The model under review builds one solid part; all positions refer to its coordinate system, in mm. Face numbers are marked on the shaded views. A direction names the side the tool comes from. Coordinates: 2 decimals unless noted, no trailing zeros. Write each loop counter-clockwise with the first axis right and the second up, starting at its lowest first coordinate (ties: lowest second). Pieces come first, ordered by that corner, then holes. Notation, with made-up numbers: (14, 60) - (54, 60) arc R18 ccw to (54, 71) - close; hole circle Ø1 at (72, -37.5). An arc over 180 degrees is marked (long way). Return JSON: item names as keys, results as strings. Group by question number.
(1) We need section D-D on z = 18. State the section outline as (x, y) points, then the cut area to 3 significant figures.
(2) We need section B-B on y = -6. State the section outline as (x, z) points, then the cut area to 3 significant figures.
(3) We need section C-C on z = -24.25. State the section outline as (x, y) points, then the cut area to 3 significant figures.
(4) Draft analysis for pull direction Y (two halves, no side actions). For the marked faces 5, 6 and 7, state which applies: released by +Y, released by -Y, zero draft, split by the parting line, or undercut.
(5) Tool access review of the marked faces 1, 2, 3 and 4: name each direction out of +Z, -Z, +X, -X, +Y, -Y from which nothing blocks a thin tool from reaching the whole face with its end or side.
(6) We need section A-A on x = 0. State the section outline as (y, z) points.
(7) To check wall thickness, follow L1, parallel to Y at x = -18.5, z = 13; L2, parallel to Y at x = 0, z = 10; L3, parallel to X at y = -10, z = 7. State the ranges of each line that lie inside material, in increasing order. Write a range as from..to.
(8) For pin 1 Ø5.5 at (x, z) = (-20.5, -24.5) entering from -Y; pin 2 Ø11.5 at (x, z) = (-20.12, 24.25) entering from +Y; pin 3 Ø4 at (y, z) = (8, -14) entering from +X, all flat-tipped, find the tip position at first contact; note any pin that passes through.
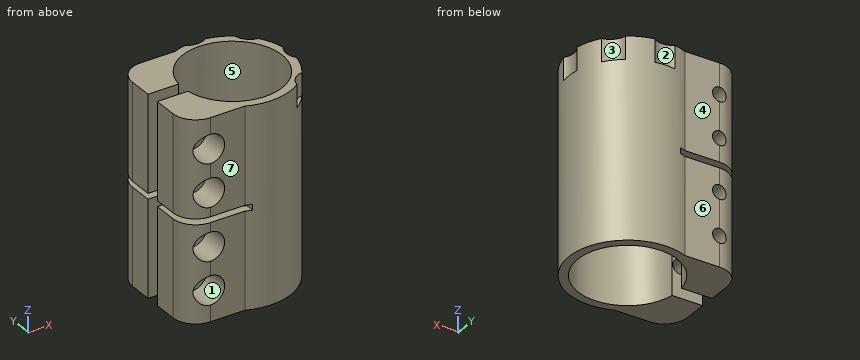
```python
from build123d import *

# Parameters (mm, degrees)
F1_DEPTH       = 35
F3_D           = 5
F3_START       = 1.7550021
F3_CBORE_D     = 10
F3_CBORE_DEPTH = 8
F4_W           = 22.4
F4_H           = 2
F5_DEPTH       = 25
F7_DEPTH       = 8


with BuildPart() as f1:
    # F0 (on Top) → F1 (new body, symmetric)
    with BuildSketch(Plane.XY):
        with BuildLine():
            ThreePointArc((-17.3192642082, 2.5086026559), (17.5, 0), (-17.3192642082, -2.5086026559))
            Line((-17.3192642082, -2.5086026559), (-28.1192642082, -2.5086026559))
            Line((-28.1192642082, -2.5086026559), (-28.1192642082, -10.9086026559))
            ThreePointArc((-28.1192642082, -10.9086026559), (-25.7761184577, -16.5654569054), (-20.1192642082, -18.9086026559))
            Line((-20.1192642082, -18.9086026559), (-7.9192642082, -18.9086026559))
            ThreePointArc((-7.9192642082, -18.9086026559), (20.5, 0), (-7.9192642082, 18.9086026559))
            Line((-7.9192642082, 18.9086026559), (-20.1192642082, 18.9086026559))
            ThreePointArc((-20.1192642082, 18.9086026559), (-25.7761184577, 16.5654569054), (-28.1192642082, 10.9086026559))
            Line((-28.1192642082, 10.9086026559), (-28.1192642082, 2.5086026559))
            Line((-28.1192642082, 2.5086026559), (-17.3192642082, 2.5086026559))
        make_face()
    extrude(amount=F1_DEPTH, both=True)

    # F3 (through all)
    # its depths count from where the whole tool has entered the part; down to there all is cleared
    with Locations(Plane.XZ.offset(18.9086026559).offset(-F3_START)):
        with Locations((-20.1192642082, 24.25), (-20.1192642082, 9.25), (-20.1192642082, -9.25), (-20.1192642082, -24.25)):
            CounterBoreHole(F3_D / 2, F3_CBORE_D / 2, F3_CBORE_DEPTH)

    # F4 (on Front) → F5 (cut, symmetric)
    with BuildSketch(Plane.XZ):
        with Locations((-16.9192642082, 0)):
            Rectangle(F4_W, F4_H)
    extrude(amount=F5_DEPTH, both=True, mode=Mode.SUBTRACT)

    # F6 (on face) → F7 (cut)
    with BuildSketch(Plane.XY.offset(35)):
        with BuildLine():
            ThreePointArc((16.8043309304, -11.7415698261), (14.4956890143, -14.4956890143), (11.7415698261, -16.8043309304))
            ThreePointArc((11.7415698261, -16.8043309304), (17.2398329286, -23.6616731318), (23.6776695297, -17.6776695297))
            ThreePointArc((23.6776695297, -17.6776695297), (21.5994018258, -13.1367427743), (16.8043309304, -11.7415698261))
        make_face()
        with BuildLine():
            ThreePointArc((16.8043309304, -11.7415698261), (13.4350288425, -13.4350288425), (11.7415698261, -16.8043309304))
            ThreePointArc((11.7415698261, -16.8043309304), (14.4956890143, -14.4956890143), (16.8043309304, -11.7415698261))
        make_face()
        with BuildLine():
            ThreePointArc((20.185, 3.5799127084), (20.5, 0), (20.185, -3.5799127084))
            ThreePointArc((20.185, -3.5799127084), (26.8854707635, -5.6960512638), (31, 0))
            ThreePointArc((31, 0), (26.8854707635, 5.6960512638), (20.185, 3.5799127084))
        make_face()
        with BuildLine():
            ThreePointArc((20.185, 3.5799127084), (19, 0), (20.185, -3.5799127084))
            ThreePointArc((20.185, -3.5799127084), (20.5, 0), (20.185, 3.5799127084))
        make_face()
        with BuildLine():
            ThreePointArc((11.7415698261, 16.8043309304), (14.4956890143, 14.4956890143), (16.8043309304, 11.7415698261))
            ThreePointArc((16.8043309304, 11.7415698261), (21.5994018258, 13.1367427743), (23.6776695297, 17.6776695297))
            ThreePointArc((23.6776695297, 17.6776695297), (17.2398329286, 23.6616731318), (11.7415698261, 16.8043309304))
        make_face()
        with BuildLine():
            ThreePointArc((11.7415698261, 16.8043309304), (13.4350288425, 13.4350288425), (16.8043309304, 11.7415698261))
            ThreePointArc((16.8043309304, 11.7415698261), (14.4956890143, 14.4956890143), (11.7415698261, 16.8043309304))
        make_face()
        with BuildLine():
            ThreePointArc((-3.5799127084, 20.185), (0, 20.5), (3.5799127084, 20.185))
            ThreePointArc((3.5799127084, 20.185), (5.3609456372, 22.305512688), (6, 25))
            ThreePointArc((6, 25), (-2.694487312, 30.3609456372), (-3.5799127084, 20.185))
        make_face()
        with BuildLine():
            ThreePointArc((-3.5799127084, 20.185), (0, 19), (3.5799127084, 20.185))
            ThreePointArc((3.5799127084, 20.185), (0, 20.5), (-3.5799127084, 20.185))
        make_face()
    extrude(amount=-F7_DEPTH, mode=Mode.SUBTRACT)


solid = f1.part
```
Ans:
{
 "1": {"outline": "(-28.12, -10.91) arc R8 ccw to (-20.12, -18.91) - (-7.92, -18.91) arc R20.5 ccw (long way) to (-7.92, 18.91) - (-20.12, 18.91) arc R8 ccw to (-28.12, 10.91) - (-28.12, 2.51) - (-17.32, 2.51) arc R17.5 cw (long way) to (-17.32, -2.51) - (-28.12, -2.51) - close", "area": "697 mm²"},
 "2": {"outline": "(-28.12, -35) - (-16.44, -35) - (-16.44, -1) - (-28.12, -1) - close; (-28.12, 1) - (-16.44, 1) - (-16.44, 35) - (-28.12, 35) - close; (16.44, -35) - (19.6, -35) - (19.6, 35) - (16.44, 35) - close; hole circle Ø5 at (-20.12, -24.25); hole circle Ø5 at (-20.12, -9.25); hole circle Ø5 at (-20.12, 9.25); hole circle Ø5 at (-20.12, 24.25)", "area": "937 mm²"},
 "3": {"outline": "(-28.12, -10.91) arc R8 ccw to (-25.12, -17.15) - (-25.12, -9.15) - (-22.62, -9.15) - (-22.62, -2.51) - (-28.12, -2.51) - close; (-28.12, 2.51) - (-22.62, 2.51) - (-22.62, 18.51) arc R8 ccw to (-28.12, 10.91) - close; (-17.62, -9.15) - (-15.12, -9.15) - (-15.12, -18.91) - (-7.92, -18.91) arc R20.5 ccw (long way) to (-7.92, 18.91) - (-17.62, 18.91) - (-17.62, 2.51) - (-17.32, 2.51) arc R17.5 cw (long way) to (-17.32, -2.51) - (-17.62, -2.51) - close", "area": "488 mm²"},
 "4": {"face 5": "undercut", "face 6": "released by +Y", "face 7": "released by -Y"},
 "5": {"face 1": "-Y", "face 2": "+Z, +Y", "face 3": "+Z, +X, +Y", "face 4": "+Z, -Z, -X, +Y"},
 "6": {"outline": "(-20.5, -35) - (-17.5, -35) - (-17.5, 35) - (-20.5, 35) - close; (17.5, -35) - (20.5, -35) - (20.5, 27) - (19, 27) - (19, 35) - (17.5, 35) - close"},
 "7": {"L1": "-9.15..-2.51, 2.51..18.91", "L2": "-20.5..-17.5, 17.5..20.5", "L3": "-28.12..-24.58, -15.65..-14.36, 14.36..17.9"},
 "8": {"pin 1": "y = -9.15", "pin 2": "y = 18.91", "pin 3": "x = 19.6"}
}
